Work out the finished part from the listing and answer in its coordinate system (mm). A direction names the side the tool comes from. Give positions to 0.01 mm unless a question says otherwise; leave off trailing zeros. Loops run counter-clockwise (first coordinate to the right, second up) from the corner with the lowest first, then second, coordinate; pieces in that order, holes last.
Autodesk Inventor part; units mm, degrees
ref_plane "YZ Plane" through (0, 0, 0) normal (1, 0, 0) x (0, 1, 0)
ref_plane "XZ Plane" through (0, 0, 0) normal (0, 1, 0) x (-1, 0, 0)
ref_plane "XY Plane" through (0, 0, 0) normal (0, 0, 1) x (1, 0, 0)
sketch "Sketch1" plane through (0, 0, 0) normal (0, 0, 1) x (1, 0, 0)
  line L0 (-12.5, 20) -> (12.5, 20)
  line L1 (12.5, 20) -> (12.5, -20)
  line L2 (12.5, -20) -> (-12.5, -20)
  line L3 (-12.5, -20) -> (-12.5, 20)
  point P0 (0, 0)
  point P1 (-12.5, 0)
  point P2 (0, 20)
  dimension "d0" = 40
  dimension "d1" = 25
extrude "Extrusion1" add sketch "Sketch1" along normal blind 15
sketch "Sketch3" plane through (0, 0, 15) normal (0, 0, -1) x (-1, 0, 0)
  line L0 (-12.5, -20) -> (-12.5, 20)
  line L1 (-12.5, -20) -> (-12.5, 20)
  line L2 (12.5, -20) -> (-12.5, -20)
  line L3 (-12.5, 20) -> (12.5, 20)
  line L4 (0, 0) -> (0, 4.9357) construction
  point P0 (-7, -14)
  point P1 (-7, 14)
  point P2 (0, -20)
  point P3 (0, 20)
  point P4 (7, -14)
  point P5 (7, 14)
  dimension "d21" = 6
  dimension "d22" = 6
  dimension "d24" = 5.5
hole "Hole1" at (7, -14, 15) at (-7, -14, 15) at (-7, 14, 15) at (7, 14, 15) direction (0, 0, -1) diameter 5 end through all counterbore diameter 10 counterbore depth 5
sketch "Sketch4" plane through (0, 0, 15) normal (0, 0, 1) x (1, 0, 0)
  line L0 (-12.5, 5) -> (12.5, 5)
  line L1 (12.5, 5) -> (12.5, -5)
  line L2 (12.5, -5) -> (-12.5, -5)
  line L3 (-12.5, -5) -> (-12.5, 5)
  line L4 (12.5, -20) -> (12.5, 20)
  line L5 (-12.5, 20) -> (-12.5, -20)
  point P0 (0, 0)
  point P1 (12.5, 0)
  dimension "d20" = 10
extrude "Extrusion3" add sketch "Sketch4" along normal blind 25
sketch "Sketch5" plane through (-12.5, 5, 15) normal (0, 1, 0) x (1, 0, 0)
  circle A0 centre (10, -13) radius 6
  line L0 (25, -25) -> (0, -25)
  line L1 (25, 0) -> (25, -25)
  circle A1 centre (10, -5) radius 1.75
  circle A2 centre (2, -13) radius 1.75
  circle A3 centre (10, -21) radius 1.75
  circle A4 centre (18, -13) radius 1.75
  point P0 (12.5, 15)
  dimension "d27" = 12
  dimension "d28" = 12
  dimension "d29" = 15
  dimension "d30" = 3.5
  dimension "d31" = 8
  dimension "d34" = 360
extrude "Extrusion4" cut sketch "Sketch5" against normal through all
fillet "Fillet2" radius 2 2 edges at (0, 5, 15) (0, -5, 15)
sketch "Sketch6" plane through (0, 0, 15) normal (0, 0, 1) x (1, 0, 0)
  line L0 (12.5, 7) -> (12.5, 20)
  line L1 (12.5, 19) -> (7, 19)
  line L2 (12.5, 9) -> (7, 9)
  circle A0 centre (7, 14) radius 5
  point P0 (0, 0)
extrude "Extrusion5" cut sketch "Sketch6" against normal up to surface (5 mm away) contours L2 A0 L1 L0
mirror "Mirror1" about plane through (0, 0, 0) normal (1, 0, 0) of "Extrusion5"
mirror "Mirror2" about plane through (0, 0, 0) normal (0, 1, 0) of "Extrusion5", "Mirror1"
properties part number "0008-10-013 Supăort Piulita Axa Z2"
Q1. Section A-A on z = 36 is taken. Give the vertices of the cut face in (x, y).
Q2. Section C-C on z = 28 is taken. Give the vertices of the cut face in (x, y).
Q3. Consider line 1 along X through (y, z) = (-14, 2); line 2 along X through (y, z) = (0.25, 28); line 3 along Z through (x, y) = (-2.5, -1.25). Determine where each line is inside the solid, lowest interval first.
Q4. Determine the mould class of faces 1 (the face through (-3.801, 0.07, 33.857)), 2 (the face through (0, 14, 15)), 3 (the face through (-2, -14, 12)) for opening direction Z: +Z half, -Z half, draft (parallel to the pull), parting line (faces both ways), or undercut.
Q5. Given pin 1 (10.5 mm diameter, centred on x = 2.5, y = 11.5, fed in from +Z); pin 2 (3 mm diameter, centred on x = 6, z = 32.5, fed in from +Y); pin 3 (11 mm diameter, centred on x = 6, y = -12.5, fed in from +Z), each flat-ended and moving along its own axis, determine where each tip first touches the part or whether it passes through.
Q6. Which of the six approach directions +Z, -Z, +X, -X, +Y, -Y give full straight-line access (tool end or side, diameter ignored) to faces 4 (the face through (-2, 14, 12)), 5 (the face through (10, -19, 13)), 6 (the face through (-2.728, 0.07, 18.265)), 7 (the face through (0, -13, 15)), 8 (the face through (-7.1, -11.5, 4.9))?
Q7. Section B-B on x = -10.5 is taken. Give the vertices of the cut face in (y, z).
Q8. Section D-D on x = -7.75 is taken. State how many separate pieces and enclosed holes the cut face has, plus the area to 3 significant figures.
Check result:
1. outline: (-12.5, -5) - (-4.25, -5) - (-4.25, 5) - (-12.5, 5) - close; (-0.75, -5) - (12.5, -5) - (12.5, 5) - (-0.75, 5) - close
2. outline: (-12.5, -5) - (-12.25, -5) - (-12.25, 5) - (-12.5, 5) - close; (-8.75, -5) - (-8.5, -5) - (-8.5, 5) - (-8.75, 5) - close; (3.5, -5) - (3.75, -5) - (3.75, 5) - (3.5, 5) - close; (7.25, -5) - (12.5, -5) - (12.5, 5) - (7.25, 5) - close
3. line 1: x = -12.5 to -9.5, -4.5 to 4.5, 9.5 to 12.5
3. line 2: x = -12.5 to -12.25, -8.75 to -8.5, 3.5 to 3.75, 7.25 to 12.5
3. line 3: z = 0 to 18.25, 21.75 to 22, 34 to 34.25, 37.75 to 40
4. face 1: undercut
4. face 2: +Z half
4. face 3: draft
5. pin 1: stops at z = 15.15
5. pin 2: stops at y = 5
5. pin 3: stops at z = 15
6. face 4: +Z, -X
6. face 5: +Z, +X
6. face 6: +Y, -Y
6. face 7: +Z, +X, -X, -Y
6. face 8: +Z, -Z
7. outline: (-20, 0) - (20, 0) - (20, 15) - (19, 15) - (19, 10) - (9, 10) - (9, 15) - (7, 15) arc R2 cw to (5, 17) - (5, 26.25) - (-5, 26.25) - (-5, 17) arc R2 cw to (-7, 15) - (-9, 15) - (-9, 10) - (-19, 10) - (-19, 15) - (-20, 15) - close; (-5, 29.75) - (5, 29.75) - (5, 40) - (-5, 40) - close
8. separate pieces: 4
8. enclosed holes: 0
8. area: 598 mm2
